Read the model definition and answer for the solid it produces. Units are mm, in the model's axes. A direction names the side the tool comes from. Coordinates: 2 decimals unless noted, no trailing zeros. Write each loop counter-clockwise with the first axis right and the second up, starting at its lowest first coordinate (ties: lowest second). Pieces come first, ordered by that corner, then holes. Notation, with made-up numbers: (-31.5, 59.25) - (15.5, 59.25) arc R24 ccw to (15.5, 87.25) - close; hole circle Ø11 at (45, 31). An arc over 180 degrees is marked (long way). Return JSON: item names as keys, results as strings.
Solid Edge part; units mm, degrees
sketch "Sketch1" plane through (0, 0, 0) normal (0, 0, -1) x (-1, 0, 0)
  circle A0 centre (8.5, -9) radius 1.6
  circle A1 centre (43.5, -9) radius 1.6
  circle A2 centre (43.5, -44) radius 1.6
  circle A3 centre (8.5, -44) radius 1.6
  arc A4 (4.2574, -39.7574) -> (4.2574, -13.2426) centre (-9, -26.5) ccw
  arc A5 (39.2574, -4.7574) -> (12.7426, -4.7574) centre (26, 8.5) cw
  arc A6 (47.7426, -13.2426) -> (47.7426, -39.7574) centre (61, -26.5) ccw
  arc A7 (39.2574, -48.2426) -> (12.7426, -48.2426) centre (26, -61.5) ccw
  arc A8 (12.7426, -48.2426) -> (4.2574, -39.7574) centre (8.5, -44) cw
  arc A9 (4.2574, -13.2426) -> (12.7426, -4.7574) centre (8.5, -9) cw
  arc A10 (39.2574, -4.7574) -> (47.7426, -13.2426) centre (43.5, -9) cw
  arc A11 (47.7426, -39.7574) -> (39.2574, -48.2426) centre (43.5, -44) cw
extrude "Protrusion1" add sketch "Sketch1" along normal blind 4
sketch "Sketch2" plane through (-26, -26.5, -4) normal (0, 0, -1) x (-1, 0, 0)
  line L0 (-19.3475, 20.7) -> (-21.195, 17.5)
  line L1 (-21.195, 17.5) -> (-19.3475, 14.3)
  line L2 (-19.3475, 14.3) -> (-15.6525, 14.3)
  line L3 (-15.6525, 14.3) -> (-13.805, 17.5)
  line L4 (-13.805, 17.5) -> (-15.6525, 20.7)
  line L5 (-15.6525, 20.7) -> (-19.3475, 20.7)
  line L6 (19.3475, 14.3) -> (21.195, 17.5)
  line L7 (21.195, 17.5) -> (19.3475, 20.7)
  line L8 (19.3475, 20.7) -> (15.6525, 20.7)
  line L9 (15.6525, 20.7) -> (13.805, 17.5)
  line L10 (13.805, 17.5) -> (15.6525, 14.3)
  line L11 (15.6525, 14.3) -> (19.3475, 14.3)
  line L12 (-19.3475, -14.3) -> (-21.195, -17.5)
  line L13 (-21.195, -17.5) -> (-19.3475, -20.7)
  line L14 (-19.3475, -20.7) -> (-15.6525, -20.7)
  line L15 (-15.6525, -20.7) -> (-13.805, -17.5)
  line L16 (-13.805, -17.5) -> (-15.6525, -14.3)
  line L17 (-15.6525, -14.3) -> (-19.3475, -14.3)
  line L18 (19.3475, -20.7) -> (21.195, -17.5)
  line L19 (21.195, -17.5) -> (19.3475, -14.3)
  line L20 (19.3475, -14.3) -> (15.6525, -14.3)
  line L21 (15.6525, -14.3) -> (13.805, -17.5)
  line L22 (13.805, -17.5) -> (15.6525, -20.7)
  line L23 (15.6525, -20.7) -> (19.3475, -20.7)
extrude "ExtrudedCutout_1" cut sketch "Sketch2" against normal blind 1
fillet "Round_1" radius 2 8 edges at (-26, -10.2487, -4) (-47.7426, -4.7574, -4) (-42.2513, -26.5, -4) (-47.7426, -48.2426, -4) (-26, -42.7513, -4) (-4.2574, -48.2426, -4) (-9.7487, -26.5, -4) (-4.2574, -4.7574, -4)
sketch "Sketch3" plane through (-26, -26.5, -4) normal (0, 0, -1) x (-1, 0, 0)
  line L0 (-10, -10) -> (10, -10)
  line L1 (10, -10) -> (10, 10)
  line L2 (10, 10) -> (-10, 10)
  line L3 (-10, 10) -> (-10, -10)
extrude "ExtrudedProtrusion_2" add sketch "Sketch3" along normal blind 20
sketch "Sketch4" plane through (-26, -26.5, -24) normal (0, 0, -1) x (-1, 0, 0)
  line L0 (-6, 10) -> (-6, -10)
  line L1 (-6, -10) -> (-2, -10)
  line L2 (-2, -10) -> (-2, 10)
  line L3 (-6, 10) -> (-2, 10)
  line L4 (2, 10) -> (2, -10)
  line L5 (2, -10) -> (6, -10)
  line L6 (6, -10) -> (6, 10)
  line L7 (6, 10) -> (2, 10)
extrude "ExtrudedCutout_2" cut sketch "Sketch4" against normal blind 20
sketch "Sketch5" plane through (-16, -26.5, -11.5) normal (1, 0, 0) x (0, -1, 0)
  arc A0 (0, 12.5) -> (-10, 2.5) centre (0, 2.5) ccw
  line L0 (-10, 2.5) -> (-11.394, 2.5)
  line L1 (-11.394, 2.5) -> (-11.394, 13.023)
  line L2 (-11.394, 13.023) -> (11.286, 13.023)
  line L3 (11.286, 13.023) -> (11.286, 2.5)
  line L4 (11.286, 2.5) -> (10, 2.5)
  arc A1 (0, 12.5) -> (10, 2.5) centre (0, 2.5) cw
extrude "ExtrudedCutout_3" cut sketch "Sketch5" against normal blind 20
fillet "Round_2" radius 2 8 edges at (-26, -16.5, -4) (-18, -16.5, -4) (-34, -16.5, -4) (-16, -26.5, -4) (-34, -36.5, -4) (-26, -36.5, -4) (-18, -36.5, -4) (-36, -26.5, -4)
sketch "Sketch6" plane through (-16, -26.5, -15) normal (1, 0, 0) x (0, 0, -1)
  circle A0 centre (-1, 0) radius 1.6
extrude "Cutout1" cut sketch "Sketch6" against normal up to vertex (20 mm away)
sketch "Sketch7" plane through (-16, -26.5, -15) normal (1, 0, 0) x (0, 0, -1)
  circle A0 centre (-1, 0) radius 3.1
extrude "ExtrudedCutout_5" cut sketch "Sketch7" against normal blind 1
sketch "Sketch8" plane through (-36, -26.5, -15) normal (-1, 0, 0) x (0, 0, 1)
  line L0 (-0.7898, 3.1) -> (-2.5796, 0)
  line L1 (-2.5796, 0) -> (-0.7898, -3.1)
  line L2 (-0.7898, -3.1) -> (2.7898, -3.1)
  line L3 (2.7898, -3.1) -> (4.5796, 0)
  line L4 (4.5796, 0) -> (2.7898, 3.1)
  line L5 (2.7898, 3.1) -> (-0.7898, 3.1)
extrude "ExtrudedCutout_6" cut sketch "Sketch8" against normal blind 1
(1) Determine the mould class of faces 6 (the face through (-35.507, -28.072, -11.328)), 7 (the face through (-17.71, -37.1, -4.57)), 8 (the face through (-5.74, -42.38, -3.51)) for opening direction Z: +Z half, -Z half, draft (parallel to the pull), parting line (faces both ways), or undercut.
Answer:
{"face 6": "undercut", "face 7": "-Z half", "face 8": "draft"}
(2) A cutting plane is placed at B-B (z = -5). Determine the outline of the cut face in (x, y).
Answer:
{"outline": "(-36.27, -36.77) - (-32, -36.77) - (-32, -16.23) - (-36.27, -16.23) - close; (-28, -36.77) - (-24, -36.77) - (-24, -16.23) - (-28, -16.23) - close; (-20, -36.77) - (-15.73, -36.77) - (-15.73, -16.23) - (-20, -16.23) - close"}
(3) A cutting plane is placed at A-A (z = -14.75). State how many separate pieces and enclosed holes the cut face has, and give its area (3 significant figures).
Answer:
{"separate pieces": "6", "enclosed holes": "0", "area": "199 mm²"}
(4) Straight lines are drawn through the part: line 1 (X direction, y = -36, z = -7.25); line 2 (Y direction, x = -26.2, z = -14); line 3 (Z direction, x = -13, y = -9). For each, find the intervals that lie inside material, in ascending order. Write a range as from..to.
Answer:
{"line 1": "-36..-32, -28..-24, -20..-16", "line 2": "-36.5..-28.1, -24.9..-16.5", "line 3": "-4..0"}
(5) Which of the six approach directions +Z, -Z, +X, -X, +Y, -Y give full straight-line access (tool end or side, diameter ignored) to faces 1 (the face through (-10, -43, -3)), 2 (the face through (-26, -16.5, -10)), 3 (the face through (-25.794, -42.752, -0.986)), 4 (the face through (-35, -28, -15)), 5 (the face through (-47.648, -4.665, -0.986))?
Answer:
{"face 1": "-Z", "face 2": "-Z, +X, -X, +Y", "face 3": "+Z, -Z, -Y", "face 4": "-X", "face 5": "+Z, -Z"}
(6) Flat-ended cylindrical pins translate along their axes: P1, Ø10, axis at y = -31.5, z = -11, coming from the +X side; P2, Ø0.5, axis at x = -7.5, z = -3.5, coming from the -Y side; P3, Ø3, axis at x = -25.5, z = -11.5, coming from the +Y side; P4, Ø3, axis at x = -43.5, y = -44, coming from the -Z side. Find the tip coordinate at first contact, or state that the pin passes through.
Answer:
{"P1": "x = -16", "P2": "y = -49.48", "P3": "y = -16.5", "P4": "through"}
